Read the model definition and answer for the solid it produces. Units are mm, in the model's axes. A direction names the side the tool comes from. Coordinates: 2 decimals unless noted, no trailing zeros. Write each loop counter-clockwise with the first axis right and the second up, starting at its lowest first coordinate (ties: lowest second). Pieces come first, ordered by that corner, then holes.
(1) Given pin 1 (1.6 mm diameter, centred on x = 0, z = 2, fed in from -Y); pin 2 (1.6 mm diameter, centred on x = -0.5, z = 1.5, fed in from +Y); pin 3 (1.5 mm diameter, centred on x = -5, z = 2.5, fed in from -Y), each flat-ended and moving along its own axis, determine where each tip first touches the part or whether it passes through.
(2) The part is cut by section C-C, the plane z = 2.1. Determine the outline of the cut face in (x, y) (1 decimal), and give its area (3 significant figures).
(3) Straight lines are drawn through the part: line 1 along Y through (x, z) = (0, 1.75); line 2 along Y through (x, z) = (0, 1.35); line 3 along X through (y, z) = (8.5, 2.15). For each, find the intervals that lie inside material, in ascending order.
(4) The part is cut by section A-A, the plane x = 0. Determine the outline of the cut face in (y, z) (1 decimal).
(5) Determine the mould class of faces 1 (the flat face through (0, 11.75, 1)), 2 (the flat face through (0, 0.934, 1)), 3 (the flat face through (0, 0, 0)), 4 (the cylindrical face through (-18.897, -14.49, 2.37)) for opening direction X: pulls with the +X half, pulls with the -X half, needs draft (parallel to the pull), parting line crosses it, or undercut.
(6) The part is cut by section D-D, the plane x = 20.5. Determine the outline of the cut face in (y, z) (1 decimal), and give its area (3 significant figures).
(7) Which of the six approach directions +Z, -Z, +X, -X, +Y, -Y give full straight-line access (tool end or side, diameter ignored) to faces 5 (the flat face through (0.788, 6, 1)), 6 (the flat face through (0, 0, 3.175)), 7 (the flat face through (-12.9, 20.2, 1.588))?
(8) The part is cut by section B-B, the plane y = 0. Determine the outline of the cut face in (x, z) (1 decimal), and give its area (3 significant figures).
```python
from build123d import *

# Parameters (mm, degrees)
F0_R         = 24.60625
F1_DEPTH     = 1.5875
F2_R         = 23.8125
F3_DEPTH     = 3.175
F6_W         = 1.888648374
F6_H         = 10.8168021543
F7_DEPTH     = 3.176
F5_R         = 2.54
F8_DEPTH     = 3.176
F4_R         = 2.54
F9_DEPTH     = 3.176
F10_C1_SIZE2 = 0.508
F10_C1_SIZE  = 0.1361181898
F10_C2_SIZE2 = 0.1361181898
F10_C2_SIZE  = 0.508
F10_C3_SIZE2 = 0.508
F10_C3_SIZE  = 0.1361181898
F10_C4_SIZE2 = 0.508
F10_C4_SIZE  = 0.1361181898
F11_SIZE2    = 0.1361181898
F11_SIZE     = 0.508
F12_SIZE2    = 0.1361181898
F12_SIZE     = 0.508


# Not quite as in the source:
# - a length typed as a fraction of an inch, garbled in the dataset ("3 / 203.2 mm" for 3/8 in), is restored


with BuildPart() as f1:
    # F0 (on Top) → F1 (new body)
    with BuildSketch(Plane.XY):
        Circle(F0_R)
    extrude(amount=F1_DEPTH)

    # F2 (on Top) → F3 (join)
    with BuildSketch(Plane.XY):
        Circle(F2_R)
    extrude(amount=F3_DEPTH)

    # F6 (on Top) → F7 (cut, through all)
    with BuildSketch(Plane.XY):
        with Locations((-0.156514463, 6.341986882)):
            Rectangle(F6_W, F6_H)
    extrude(amount=F7_DEPTH, mode=Mode.SUBTRACT)

    # F5 (on Top) → F8 (cut, through all)
    with BuildSketch(Plane.XY):
        with Locations((6.0491965251, -7.797766786)):
            Circle(F5_R)
    extrude(amount=F8_DEPTH, mode=Mode.SUBTRACT)

    # F4 (on Top) → F9 (cut, through all)
    with BuildSketch(Plane.XY):
        with Locations((-6.5096618418, -7.5848015673)):
            Circle(F4_R)
    extrude(amount=F9_DEPTH, mode=Mode.SUBTRACT)

    # F10: chamfer of 0.508 x 0.1361181898 on 4 edges, made by hand

    # F10_c1
    f10_c1_edges = [f1.edges().sort_by_distance(p)[0] for p in [
        (-1.10083865, 6.341986882, 0),
    ]]
    f10_c1_side = f1.faces().sort_by_distance((-1.1035610138, 6.341986882, 0))[0]
    chamfer(f10_c1_edges, length=F10_C1_SIZE, length2=F10_C1_SIZE2, reference=f10_c1_side)

    # F10_c2
    f10_c2_edges = [f1.edges().sort_by_distance(p)[0] for p in [
        (-0.156514463, 0.9335858049, 3.175),
    ]]
    f10_c2_side = f1.faces().sort_by_distance((-0.156514463, 0.9335858049, 3.1722776362))[0]
    chamfer(f10_c2_edges, length=F10_C2_SIZE, length2=F10_C2_SIZE2, reference=f10_c2_side)

    # F10_c3
    f10_c3_edges = [f1.edges().sort_by_distance(p)[0] for p in [
        (0.787809724, 6.341986882, 3.175),
    ]]
    f10_c3_side = f1.faces().sort_by_distance((0.787809724, 6.341986882, 3.1722776362))[0]
    chamfer(f10_c3_edges, length=F10_C3_SIZE, length2=F10_C3_SIZE2, reference=f10_c3_side)

    # F10_c4
    f10_c4_edges = [f1.edges().sort_by_distance(p)[0] for p in [
        (-0.156514463, 11.7503879592, 3.175),
    ]]
    f10_c4_side = f1.faces().sort_by_distance((-0.156514463, 11.7503879592, 3.1722776362))[0]
    chamfer(f10_c4_edges, length=F10_C4_SIZE, length2=F10_C4_SIZE2, reference=f10_c4_side)

    # F11
    f11_edges = [f1.edges().sort_by_distance(p)[0] for p in [
        (-9.049662, -7.584802, 3.175),
    ]]
    chamfer(f11_edges, length=F11_SIZE, length2=F11_SIZE2)

    # F12
    f12_edges = [f1.edges().sort_by_distance(p)[0] for p in [
        (3.509197, -7.797767, 3.175),
    ]]
    chamfer(f12_edges, length=F12_SIZE, length2=F12_SIZE2)


solid = f1.part
```
Computed:
1. pin 1: stops at y = -24.61
1. pin 2: stops at y = 24.61
1. pin 3: stops at y = -23.43
2. outline: circle Ø47.6 at (0, 0); hole circle Ø5.1 at (-6.5, -7.6); hole (-1.1, 0.9) - (0.8, 0.9) - (0.8, 11.8) - (-1.1, 11.8) - close; hole circle Ø5.1 at (6, -7.8)
2. area: 1,720 mm2
3. line 1: y = -23.81 to 0.93, 11.75 to 23.81
3. line 2: y = -24.61 to 0.93, 11.75 to 24.61
3. line 3: x = -22.24 to -1.1, 0.79 to 22.24
4. outline: (-24.6, 0) - (0.9, 0) - (0.9, 2.7) - (0.8, 3.2) - (-23.8, 3.2) - (-23.8, 1.6) - (-24.6, 1.6) - close; (11.8, 0) - (24.6, 0) - (24.6, 1.6) - (23.8, 1.6) - (23.8, 3.2) - (12.3, 3.2) - (11.8, 3) - close
5. face 1: undercut
5. face 2: undercut
5. face 3: needs draft
5. face 4: parting line crosses it
6. outline: (-13.6, 0) - (13.6, 0) - (13.6, 1.6) - (12.1, 1.6) - (12.1, 3.2) - (-12.1, 3.2) - (-12.1, 1.6) - (-13.6, 1.6) - close
6. area: 81.7 mm2
7. face 5: +Z, -Z
7. face 6: +Z, +X, -X, +Y, -Y
7. face 7: +Z
8. outline: (-24.6, 0) - (24.6, 0) - (24.6, 1.6) - (23.8, 1.6) - (23.8, 3.2) - (-23.8, 3.2) - (-23.8, 1.6) - (-24.6, 1.6) - close
8. area: 154 mm2
